The listing builds one solid part. Answer for the finished solid, in the listing's coordinates (mm). Face numbers are marked on the shaded views. A direction names the side the tool comes from. Give positions to 0.01 mm unless a question says otherwise; leave off trailing zeros. Order: outer loops, then holes, each group sorted by start corner. A loop starts at its lowest first (then second) coordinate and runs counter-clockwise, first axis right, second up. Notation, with made-up numbers: (63, -20) - (86, -20) arc R23 cw to (86, 4) - close; hole circle Ø8 at (-23.75, -19). An arc over 180 degrees is marked (long way). Use a Markdown table: item, result. Add a question column.
1) Flat-ended cylindrical pins translate along their axes: pin 1 (11.5 mm diameter, centred on x = 3.5, y = -85.5, fed in from +Z); pin 2 (6.5 mm diameter, centred on x = 22.52, y = 13, fed in from +Z); pin 3 (4 mm diameter, centred on x = 16, y = -37, fed in from +Z); pin 4 (1.5 mm diameter, centred on y = -62, z = 6.5, fed in from +X). Find the tip coordinate at first contact, or state that the pin passes through.
2) Find section B-B, the plane z = 12.25. State how many separate pieces and enclosed holes the cut face has, plus the area to 3 significant figures.
3) For the marked faces 1, 2 and 3, determine the directions among +Z, -Z, +X, -X, +Y, -Y from which every point of the face is accessible in a straight line to the end or side of a thin tool.
4) Straight lines are drawn through the part: line 1 (Y direction, x = 0, z = 8); line 2 (X direction, y = -49.5, z = 5.75); line 3 (X direction, y = -85, z = 7.25). For each, find the intervals that lie inside material, in ascending order.
5) Find section A-A, the plane x = -42. Determine the outline of the cut face in (y, z).
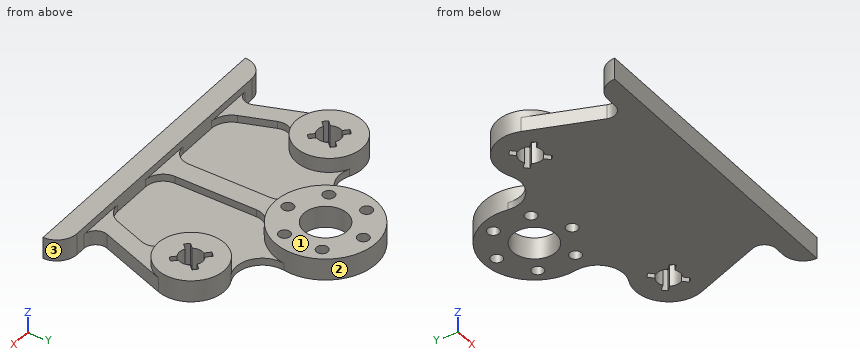
from build123d import *

# Parameters (mm, degrees)
EXTRUDE_1_DEPTH   = 5
EXTRUDE_1_2_DEPTH = 5
SKETCH_1_3_R      = 35
SKETCH_1_3_R_2    = 4
SKETCH_1_3_R_3    = 15
SKETCH_1_3_R_4    = 23
EXTRUDE_2_DEPTH   = 15
EXTRUDE_3_DEPTH   = 10


with BuildPart() as part:
    # Sketch 1 → Extrude 1 (new body)
    with BuildSketch(Plane.XY):
        with BuildLine():
            ThreePointArc((34.601893463, -5.263930923), (27.803487019, -21.259494575), (14.14893617, -32.012616345))
            ThreePointArc((14.14893617, -32.012616345), (8.944833021, -36.439048645), (7, -42.98837052))
            Line((7, -42.98837052), (7, -99))
            ThreePointArc((7, -99), (10.514718626, -107.485281374), (19, -111))
            Line((19, -111), (47.466246321, -111))
            ThreePointArc((47.466246321, -111), (55.456771013, -108.495717253), (60.588648114, -101.878787879))
            Line((60.588648114, -101.878787879), (68.815739838, -79.750503994))
            ThreePointArc((68.815739838, -79.750503994), (68.470432654, -71.964706785), (62.641809124, -66.791214446))
            ThreePointArc((62.641809124, -66.791214446), (47.040096479, -46.357508857), (60.125232147, -24.227687662))
            ThreePointArc((60.125232147, -24.227687662), (41.662021509, -22.419519283), (34.601893463, -5.263930923))
        make_face()
    extrude(amount=EXTRUDE_1_DEPTH)



with BuildPart() as body_2:
    # Sketch 1 → Extrude 1 2 (new body)
    with BuildSketch(Plane.XY):
        with BuildLine():
            Line((-7, -99), (-7, -42.98837052))
            ThreePointArc((-7, -42.98837052), (-8.944833021, -36.439048645), (-14.14893617, -32.012616345))
            ThreePointArc((-14.14893617, -32.012616345), (-27.803487019, -21.259494575), (-34.601893463, -5.263930923))
            ThreePointArc((-34.601893463, -5.263930923), (-41.662021509, -22.419519283), (-60.125232147, -24.227687662))
            ThreePointArc((-60.125232147, -24.227687662), (-50.556239296, -32.714228974), (-47, -45))
            ThreePointArc((-47, -45), (-51.315268397, -58.411964991), (-62.641809124, -66.791214446))
            ThreePointArc((-62.641809124, -66.791214446), (-68.470432654, -71.964706785), (-68.815739838, -79.750503994))
            Line((-68.815739838, -79.750503994), (-60.588648114, -101.878787879))
            ThreePointArc((-60.588648114, -101.878787879), (-55.456771013, -108.495717253), (-47.466246321, -111))
            Line((-47.466246321, -111), (-19, -111))
            ThreePointArc((-19, -111), (-10.514718626, -107.485281374), (-7, -99))
        make_face()
    extrude(amount=EXTRUDE_1_2_DEPTH)


with BuildPart() as part_1:
    add(part.part)

    add(body_2.part)  # Extrude 2 merges body 2
    # Sketch 1_3 → Extrude 2 (add)
    # profile 1 of 4: a face of its own
    with BuildSketch(Plane.XY):
        with Locations(Location((0, 0, 0), (0, 0, 188.649993466))):
            Circle(SKETCH_1_3_R)
        with Locations((-22.516660498, 13)):
            Circle(SKETCH_1_3_R_2, mode=Mode.SUBTRACT)
        with Locations((-22.516660498, -13)):
            Circle(SKETCH_1_3_R_2, mode=Mode.SUBTRACT)
        with Locations((0, -26)):
            Circle(SKETCH_1_3_R_2, mode=Mode.SUBTRACT)
        with Locations((22.516660498, -13)):
            Circle(SKETCH_1_3_R_2, mode=Mode.SUBTRACT)
        with Locations((22.516660498, 13)):
            Circle(SKETCH_1_3_R_2, mode=Mode.SUBTRACT)
        with Locations((0, 26)):
            Circle(SKETCH_1_3_R_2, mode=Mode.SUBTRACT)
        Circle(SKETCH_1_3_R_3, mode=Mode.SUBTRACT)
    # profile 2 of 4: a face of its own
    with BuildSketch(Plane.XY):
        with Locations(Location((-70, -45, 0), (0, 0, 288.658168076))):
            Circle(SKETCH_1_3_R_4)
        with BuildLine():
            ThreePointArc((-76.891439137, -40.936987987), (-78, -45), (-76.891439137, -49.063012013))
            Line((-76.891439137, -49.063012013), (-80.139177746, -52.310750621))
            ThreePointArc((-80.139177746, -52.310750621), (-78.838834765, -53.838834765), (-77.310750621, -55.139177746))
            Line((-77.310750621, -55.139177746), (-74.063012013, -51.891439137))
            ThreePointArc((-74.063012013, -51.891439137), (-70, -53), (-65.936987987, -51.891439137))
            Line((-65.936987987, -51.891439137), (-62.689249379, -55.139177746))
            ThreePointArc((-62.689249379, -55.139177746), (-61.161165235, -53.838834765), (-59.860822254, -52.310750621))
            Line((-59.860822254, -52.310750621), (-63.108560863, -49.063012013))
            ThreePointArc((-63.108560863, -49.063012013), (-62, -45), (-63.108560863, -40.936987987))
            Line((-63.108560863, -40.936987987), (-59.860822254, -37.689249379))
            ThreePointArc((-59.860822254, -37.689249379), (-61.161165235, -36.161165235), (-62.689249379, -34.860822254))
            Line((-62.689249379, -34.860822254), (-65.936987987, -38.108560863))
            ThreePointArc((-65.936987987, -38.108560863), (-70, -37), (-74.063012013, -38.108560863))
            Line((-74.063012013, -38.108560863), (-77.310750621, -34.860822254))
            ThreePointArc((-77.310750621, -34.860822254), (-78.838834765, -36.161165235), (-80.139177746, -37.689249379))
            Line((-80.139177746, -37.689249379), (-76.891439137, -40.936987987))
        make_face(mode=Mode.SUBTRACT)
    # profile 3 of 4: a face of its own
    with BuildSketch(Plane.XY):
        with Locations(Location((70, -45, 0), (0, 0, 115.42553834))):
            Circle(SKETCH_1_3_R_4)
        with BuildLine():
            Line((59.860822254, -37.689249379), (63.108560863, -40.936987987))
            ThreePointArc((63.108560863, -40.936987987), (62, -45), (63.108560863, -49.063012013))
            Line((63.108560863, -49.063012013), (59.860822254, -52.310750621))
            ThreePointArc((59.860822254, -52.310750621), (61.161165235, -53.838834765), (62.689249379, -55.139177746))
            Line((62.689249379, -55.139177746), (65.936987987, -51.891439137))
            ThreePointArc((65.936987987, -51.891439137), (70, -53), (74.063012013, -51.891439137))
            Line((74.063012013, -51.891439137), (77.310750621, -55.139177746))
            ThreePointArc((77.310750621, -55.139177746), (78.838834765, -53.838834765), (80.139177746, -52.310750621))
            Line((80.139177746, -52.310750621), (76.891439137, -49.063012013))
            ThreePointArc((76.891439137, -49.063012013), (78, -45), (76.891439137, -40.936987987))
            Line((76.891439137, -40.936987987), (80.139177746, -37.689249379))
            ThreePointArc((80.139177746, -37.689249379), (78.838834765, -36.161165235), (77.310750621, -34.860822254))
            Line((77.310750621, -34.860822254), (74.063012013, -38.108560863))
            ThreePointArc((74.063012013, -38.108560863), (70, -37), (65.936987987, -38.108560863))
            Line((65.936987987, -38.108560863), (62.689249379, -34.860822254))
            ThreePointArc((62.689249379, -34.860822254), (61.161165235, -36.161165235), (59.860822254, -37.689249379))
        make_face(mode=Mode.SUBTRACT)
    # profile 4 of 4: a face of its own
    with BuildSketch(Plane.XY):
        with BuildLine():
            ThreePointArc((88.5, -111), (98.399494937, -115.100505063), (102.5, -125))
            Line((102.5, -125), (-102.5, -125))
            ThreePointArc((-102.5, -125), (-98.399494937, -115.100505063), (-88.5, -111))
            Line((-88.5, -111), (88.5, -111))
        make_face()
    extrude(amount=EXTRUDE_2_DEPTH)

    # Sketch 1_4 → Extrude 3 (add)
    with BuildSketch(Plane.XY):
        with BuildLine():
            Line((-81.509349081, -111), (-47.466246321, -111))
            ThreePointArc((-47.466246321, -111), (-55.456771013, -108.495717253), (-60.588648114, -101.878787879))
            Line((-60.588648114, -101.878787879), (-68.815739838, -79.750503994))
            ThreePointArc((-68.815739838, -79.750503994), (-68.470432654, -71.964706785), (-62.641809124, -66.791214446))
            ThreePointArc((-62.641809124, -66.791214446), (-79.892182066, -65.764024994), (-91.558231518, -53.015151515))
            Line((-91.558231518, -53.015151515), (-74.010833771, -100.212121212))
            ThreePointArc((-74.010833771, -100.212121212), (-74.940367794, -107.56601411), (-81.509349081, -111))
        make_face()
        with BuildLine():
            ThreePointArc((-14.14893617, -32.012616345), (-8.944833021, -36.439048645), (-7, -42.98837052))
            Line((-7, -42.98837052), (-7, -99))
            ThreePointArc((-7, -99), (-10.514718626, -107.485281374), (-19, -111))
            Line((-19, -111), (19, -111))
            ThreePointArc((19, -111), (10.514718626, -107.485281374), (7, -99))
            Line((7, -99), (7, -42.98837052))
            ThreePointArc((7, -42.98837052), (8.944833021, -36.439048645), (14.14893617, -32.012616345))
            ThreePointArc((14.14893617, -32.012616345), (0, -35), (-14.14893617, -32.012616345))
        make_face()
        with BuildLine():
            ThreePointArc((60.588648114, -101.878787879), (55.456771013, -108.495717253), (47.466246321, -111))
            Line((47.466246321, -111), (81.509349081, -111))
            ThreePointArc((81.509349081, -111), (74.940367794, -107.56601411), (74.010833771, -100.212121212))
            Line((74.010833771, -100.212121212), (91.558231518, -53.015151515))
            ThreePointArc((91.558231518, -53.015151515), (79.892182066, -65.764024994), (62.641809124, -66.791214446))
            ThreePointArc((62.641809124, -66.791214446), (68.470432654, -71.964706785), (68.815739838, -79.750503994))
            Line((68.815739838, -79.750503994), (60.588648114, -101.878787879))
        make_face()
    extrude(amount=EXTRUDE_3_DEPTH)


solid = part_1.part
The answers:
| question | item | result |
|---|---|---|
| 1 | pin 1 | z = 10 |
| 1 | pin 2 | through |
| 1 | pin 3 | z = 5 |
| 1 | pin 4 | x = 88.5 |
| 2 | separate pieces | 4 |
| 2 | enclosed holes | 9 |
| 2 | area | 8,400 mm2 |
| 3 | face 1 | +Z, +X, -X, +Y, -Y |
| 3 | face 2 | +Z |
| 3 | face 3 | +Z, -Z, +X |
| 4 | line 1 | -125 to -30, -22 to -15, 15 to 22, 30 to 35 |
| 4 | line 2 | -92.56 to -77.33, -62.67 to -47.44, -7 to 7, 47.44 to 62.67, 77.33 to 92.56 |
| 4 | line 3 | -79.67 to -66.86, -7 to 7, 66.86 to 79.67 |
| 5 | outline | (-125, 0) - (-22.66, 0) - (-22.66, 5) - (-111, 5) - (-111, 15) - (-125, 15) - close |
